```python
from build123d import *

# Parameters (mm, degrees)
SKETCH1_W            = 102
SKETCH1_H            = 77
BOSS_EXTRUDE1_DEPTH  = 2
BOSS_EXTRUDE2_DEPTH  = 27.6
FILLET1_R            = 4
FILLET3_R            = 4
M3_CLEARANCE_HOLE1_D = 3.4
BOSS_EXTRUDE3_DEPTH  = 3
FILLET4_R            = 4
SKETCH6_W            = 14
SKETCH6_H            = 17.55
CUT_EXTRUDE1_DEPTH   = 5
SKETCH8_W            = 46.1
SKETCH8_H            = 8
CUT_EXTRUDE3_DEPTH   = 5
SKETCH9_W            = 3.59
SKETCH9_H            = 17.24
CUT_EXTRUDE4_DEPTH   = 5
FILLET5_R            = 2


with BuildPart() as part:
    # Sketch1 → Boss-Extrude1 (new body)
    with BuildSketch(Plane.XY):
        with BuildLine():
            Line((5.656854249, 0), (112.343145751, 0))
            Line((112.343145751, 0), (119.414213562, -7.071067812))
            ThreePointArc((119.414213562, -7.071067812), (125.071067812, -7.071067812), (125.071067812, -1.414213562))
            Line((125.071067812, -1.414213562), (118, 5.656854249))
            Line((118, 5.656854249), (118, 87.343145751))
            Line((118, 87.343145751), (125.071067812, 94.414213562))
            ThreePointArc((125.071067812, 94.414213562), (125.071067812, 100.071067812), (119.414213562, 100.071067812))
            Line((119.414213562, 100.071067812), (112.343145751, 93))
            Line((112.343145751, 93), (5.656854249, 93))
            Line((5.656854249, 93), (-1.414213562, 100.071067812))
            ThreePointArc((-1.414213562, 100.071067812), (-7.071067812, 100.071067812), (-7.071067812, 94.414213562))
            Line((-7.071067812, 94.414213562), (0, 87.343145751))
            Line((0, 87.343145751), (0, 5.656854249))
            Line((0, 5.656854249), (-7.071067812, -1.414213562))
            ThreePointArc((-7.071067812, -1.414213562), (-7.071067812, -7.071067812), (-1.414213562, -7.071067812))
            Line((-1.414213562, -7.071067812), (5.656854249, 0))
        make_face()
        with Locations((59, 46.5)):
            Rectangle(SKETCH1_W, SKETCH1_H, mode=Mode.SUBTRACT)
    extrude(amount=BOSS_EXTRUDE1_DEPTH)

    # Sketch2 → Boss-Extrude2 (add)
    with BuildSketch(Plane.XY.offset(2)):
        Polygon((0, 93), (0, 0), (118, 0), (118, 93), (115.3, 93), (115.3, 2.7), (2.7, 2.7), (2.7, 93), align=None)
    extrude(amount=BOSS_EXTRUDE2_DEPTH)

    # Fillet1
    fillet1_edges = [part.edges().sort_by_distance(p)[0] for p in [
        (8, 85, 1),
        (8, 8, 1),
        (110, 8, 1),
        (110, 85, 1),
    ]]
    fillet(fillet1_edges, radius=FILLET1_R)

    # Fillet3
    fillet3_edges = [part.edges().sort_by_distance(p)[0] for p in [
        (112.343145751, 0, 1),
        (5.656854249, 0, 1),
        (0, 5.656854249, 1),
        (0, 87.343145751, 1),
        (5.656854249, 93, 1),
        (112.343145751, 93, 1),
        (118, 87.343145751, 1),
        (118, 5.656854249, 1),
    ]]
    fillet(fillet3_edges, radius=FILLET3_R)

    # M3 Clearance Hole1 (through all)
    with Locations(Plane.XY.offset(2)):
        with Locations((-3.972495555, 96.92383124), (121.87433229, 96.92383124), (121.87433229, -3.91357469), (-3.972495555, -3.91357469)):
            Hole(M3_CLEARANCE_HOLE1_D / 2)

    # Sketch5 → Boss-Extrude3 (add)
    with BuildSketch(Plane.XY.offset(29.6)):
        Polygon((0, 93), (5.7, 93), (5.7, 5.7), (112.3, 5.7), (112.3, 93), (118, 93), (118, 0), (0, 0), align=None)
    extrude(amount=BOSS_EXTRUDE3_DEPTH)

    # Fillet4
    fillet4_edges = [part.edges().sort_by_distance(p)[0] for p in [
        (0, 0, 17.3),
        (118, 0, 17.3),
        (118, 93, 17.3),
        (0, 93, 17.3),
        (59, 0, 32.6),
        (118, 46.5, 32.6),
        (0, 46.5, 32.6),
    ]]
    fillet(fillet4_edges, radius=FILLET4_R)

    # Sketch6 → Cut-Extrude1 (cut)
    with BuildSketch(Plane.ZY):
        with Locations((17.37699989, 54.836937287)):
            Rectangle(SKETCH6_W, SKETCH6_H)
    extrude(amount=-CUT_EXTRUDE1_DEPTH, mode=Mode.SUBTRACT)

    # Sketch8 → Cut-Extrude3 (cut)
    with BuildSketch(Plane.XZ):
        with Locations((39.295, 13.26259989)):
            Rectangle(SKETCH8_W, SKETCH8_H)
    extrude(amount=-CUT_EXTRUDE3_DEPTH, mode=Mode.SUBTRACT)

    # Sketch9 → Cut-Extrude4 (cut)
    with BuildSketch(Plane(origin=(118, 0, 0), x_dir=(0, 0, -1), z_dir=(1, 0, 0))):
        with Locations((-11.55759989, 69.828337287)):
            Rectangle(SKETCH9_W, SKETCH9_H)
    extrude(amount=-CUT_EXTRUDE4_DEPTH, mode=Mode.SUBTRACT)

    # Fillet5
    fillet5_edges = [part.edges().sort_by_distance(p)[0] for p in [
        (16.245, 1.35, 9.26259989),
        (16.245, 1.35, 17.26259989),
        (62.345, 1.35, 17.26259989),
        (62.345, 1.35, 9.26259989),
    ]]
    fillet(fillet5_edges, radius=FILLET5_R)


solid = part.part
```
Part model, mm, in its own coordinate system. A direction names the side the tool comes from. Coordinates: 2 decimals unless noted, no trailing zeros. Order: outer loops, then holes, each group sorted by start corner. A loop starts at its lowest first (then second) coordinate and runs counter-clockwise, first axis right, second up. Notation, with made-up numbers: (68, -18.5) -> (76, -18.5) arc R25 cw to (76, 9.5) -> close; hole circle Ø3 at (29, -17). An arc over 180 degrees is marked (long way). Put each result on its own line as item: value. Start each with the question number.
(1) Band-saw the part on D-D (y = 58.5). Give the cut face in (x, z), then the cut area to 3 significant figures.
(2) Band-saw the part on B-B (y = 30.5). Give the cut face in (x, z).
(3) Band-saw the part on C-C (x = 72). Give the cut face in (y, z).
(4) Mould opens along Z. For faces 1 (the face through (2.7, 47, 9)), 2 (the face through (1.141, 49.123, 31.397)), 3 (the face through (9.141, 83.797, 1.014)) say: pulls with the +Z half, pulls with the -Z half, needs draft (parallel to the pull), parting line crosses it, or undercut.
(5) Probe line 1 along X through (y, z) = (8.5, 17.5); line 2 along Z through (x, y) = (73.5, 5.5); line 3 along Y through (x, z) = (76, 5). List the from-to ranges inside material, lowest first. Write a range as [from, to].
(6) Which spindle directions (+Z, -Z, +X, -X, +Y, -Y) get a long thin tool onto all of the face, cutting with end or side? Do faces 4 (the face through (39, 1, 9.263)), 5 (the face through (1, 46.062, 17)), 6 (the face through (58, 5.7, 31)). Say none if no direction does.
(7) Pin check, flat tips, straight feed: pin 1 Ø8 at (x, z) = (44, 4.5) entering from +Y; pin 2 Ø0.8 at (x, y) = (116.5, 66) entering from +Z; pin 3 Ø1.5 at (x, z) = (87.5, 29) entering from -Y; pin 4 Ø2.5 at (x, y) = (121.87, 96.92) entering from -Z. Stop position of each tip, or through.
(8) Band-saw the part on A-A (x = 23.5). Give the cut face in (y, z).
Determined:
1. outline: (0, 0) -> (8, 0) -> (8, 2) -> (2.7, 2) -> (2.7, 10.38) -> (0, 10.38) -> close; (0, 24.38) -> (2.7, 24.38) -> (2.7, 29.6) -> (5.7, 29.6) -> (5.7, 32.6) -> (4, 32.6) arc R4 ccw to (0, 28.6) -> close; (110, 0) -> (118, 0) -> (118, 28.6) arc R4 ccw to (114, 32.6) -> (112.3, 32.6) -> (112.3, 29.6) -> (115.3, 29.6) -> (115.3, 2) -> (110, 2) -> close
1. area: 171 mm²
2. outline: (0, 0) -> (8, 0) -> (8, 2) -> (2.7, 2) -> (2.7, 29.6) -> (5.7, 29.6) -> (5.7, 32.6) -> (4, 32.6) arc R4 ccw to (0, 28.6) -> close; (110, 0) -> (118, 0) -> (118, 28.6) arc R4 ccw to (114, 32.6) -> (112.3, 32.6) -> (112.3, 29.6) -> (115.3, 29.6) -> (115.3, 2) -> (110, 2) -> close
3. outline: (0, 0) -> (8, 0) -> (8, 2) -> (2.7, 2) -> (2.7, 29.6) -> (5.7, 29.6) -> (5.7, 32.6) -> (4, 32.6) arc R4 ccw to (0, 28.6) -> close; (85, 0) -> (93, 0) -> (93, 2) -> (85, 2) -> close
4. face 1: undercut
4. face 2: pulls with the +Z half
4. face 3: needs draft
5. line 1: x = [0, 2.7], [115.3, 118]
5. line 2: z = [0, 2], [29.6, 32.6]
5. line 3: y = [0, 2.7]
6. face 4: +Y, -Y
6. face 5: -X
6. face 6: +Z, +Y
7. pin 1: stops at y = 93
7. pin 2: stops at z = 32
7. pin 3: stops at y = 0
7. pin 4: passes through
8. outline: (0, 0) -> (8, 0) -> (8, 2) -> (2.7, 2) -> (2.7, 9.26) -> (0, 9.26) -> close; (0, 17.26) -> (2.7, 17.26) -> (2.7, 29.6) -> (5.7, 29.6) -> (5.7, 32.6) -> (4, 32.6) arc R4 ccw to (0, 28.6) -> close; (85, 0) -> (93, 0) -> (93, 2) -> (85, 2) -> close
